Can you work these out from the model? Positions are in its coordinate system, mm. A direction names the side the tool comes from. Give positions to 0.01 mm unless a question says otherwise; leave off trailing zeros. Order: outer loops, then holes, each group sorted by start corner. A loop starts at its lowest first (then second) coordinate and runs counter-clockwise, first axis right, second up. Notation, with made-up numbers: M 43.5,-24 L 69.5,-24 A29 ccw 69.5,1 Z; hole C -25.75,64 d1. An arc over 180 degrees is marked long. Use one line per item in the form item = value. Start each with the question number.
1. I want a section at A-A, the plane z = -35. List the corners of the cut face in (x, y) for me (3 decimals), and give its area (3 significant figures).
2. I want a section at B-B, the plane y = 0.75. List the corners of the cut face in (x, z) for me.
3. For faces 4 (the face through (-9, 1, 3.5)), 5 (the face through (-15, 1, -43)), 6 (the face through (-40, 1, -34)), 7 (the face through (-22, 1, -6)), 8 (the face through (-6, 1, -24)), which set-ups out of +Z, -Z, +X, -X, +Y, -Y let a thin tool reach every point of the face, with its end or its side?
4. I need wall thicknesses on L1, parallel to Z at x = 0, y = 0.9; L2, parallel to Z at x = -3, y = 0.1; L3, parallel to Z at x = -17, y = 1.15. Which ranges of each line are inside material? Lowest first, please.
5. Will these pins go through, and if not, where does the flat tip stop? P1, Ø1.5, axis at x = -24.5, z = -45.5, coming from the -Y side; P2, Ø0.5, axis at y = 1, z = -41, coming from the +X side; P3, Ø0.5, axis at y = 1, z = -8, coming from the -X side.
6. I want a section at C-C, the plane z = -24. List the corners of the cut face in (x, y) for me (3 decimals).
7. We'd pull the mould along X, two halves only. Please class faces 1 (the face through (-39.14, 0.8, -51.6)), 2 (the face through (-18, 0, -24)), 3 (the face through (-11.73, 0.8, -22.78)): +X half, -X half, draft (parallel to the pull), parting line (faces both ways), or undercut.
8. I want a section at D-D, the plane x = -4. List the corners of the cut face in (y, z) for me (3 decimals).
Autodesk Inventor part; units mm, degrees
ref_plane "YZ Plane" through (0, 0, 0) normal (1, 0, 0) x (0, 1, 0)
ref_plane "XZ Plane" through (0, 0, 0) normal (0, 1, 0) x (-1, 0, 0)
ref_plane "XY Plane" through (0, 0, 0) normal (0, 0, 1) x (1, 0, 0)
sketch "Sketch1" plane through (0, 0, 0) normal (0, 1, 0) x (-1, 0, 0)
  circle A0 centre (0, 0) radius 1.3
  circle A1 centre (0, -49) radius 1.3
  arc A2 (0, 3.5) -> (0, -3.5) centre (0, 0) ccw
  arc A3 (0, -45.5) -> (0, -52.5) centre (0, -49) ccw
  line L0 (0, 3.5) -> (19, 3.5)
  line L1 (22, 0.5) -> (22, -13.5)
  line L2 (25, -16.5) -> (37, -16.5)
  line L3 (40, -19.5) -> (40, -49.5)
  line L4 (37, -52.5) -> (0, -52.5)
  line L5 (0, -3.5) -> (3, -3.5)
  line L6 (6, -6.5) -> (6, -42.5)
  line L7 (3, -45.5) -> (0, -45.5)
  arc A4 (6, -6.5) -> (3, -3.5) centre (3, -6.5) ccw
  arc A5 (22, 0.5) -> (19, 3.5) centre (19, 0.5) ccw
  arc A6 (22, -13.5) -> (25, -16.5) centre (25, -13.5) ccw
  arc A7 (40, -19.5) -> (37, -16.5) centre (37, -19.5) ccw
  arc A8 (37, -52.5) -> (40, -49.5) centre (37, -49.5) ccw
  arc A9 (3, -45.5) -> (6, -42.5) centre (3, -42.5) ccw
  circle A10 centre (12, -24) radius 1.25
  circle A11 centre (12, -45.5) radius 1.25
  circle A12 centre (24.5, -45.5) radius 1.25
  circle A13 centre (24.5, -24) radius 1.25
  line L8 (28.5, -30) -> (12, -30)
  line L9 (12, -30) -> (12, -43)
  line L10 (12, -43) -> (19, -43)
  line L11 (19, -43) -> (19, -39.5)
  line L12 (19, -39.5) -> (28.5, -39.5)
  line L13 (28.5, -39.5) -> (28.5, -30)
  line L14 (28.5, -34.75) -> (12, -34.75) construction
  point P0 (22, 3.5)
  point P1 (22, -16.5)
  point P2 (40, -52.5)
  dimension "d0" = 49
  dimension "d1" = 2.6
  dimension "d2" = 7
  dimension "d3" = 22
  dimension "d4" = 20
  dimension "d5" = 40
  dimension "d6" = 6
  dimension "d7" = 3
  dimension "d14" = 2.5
  dimension "d15" = 12.5
  dimension "d16" = 12
  dimension "d17" = 9.5
  dimension "d18" = 3.5
  dimension "d19" = 7
  dimension "d20" = 21.5
  dimension "d21" = 7
extrude "Extrusion1" add sketch "Sketch1" along normal blind 1.615
properties part number "freestanding_cam_mount"
Check result:
q1.outline = M -40,0 L -28.5,0 L -28.5,1.615 L -40,1.615 Z; M -12,0 L -6,0 L -6,1.615 L -12,1.615 Z
q1.area = 28.3 mm2
q2.outline = M -40,-49.5 A3 ccw -37,-52.5 L 0,-52.5 A3.5 ccw 0,-45.5 L -3,-45.5 A3 cw -6,-42.5 L -6,-6.5 A3 cw -3,-3.5 L 0,-3.5 A3.5 ccw 0,3.5 L -19,3.5 A3 ccw -22,0.5 L -22,-13.5 A3 cw -25,-16.5 L -37,-16.5 A3 ccw -40,-19.5 Z; hole M -28.5,-39.5 L -19,-39.5 L -19,-43 L -12,-43 L -12,-30 L -28.5,-30 Z; hole C -24.5,-45.5 d2.5; hole C -24.5,-24 d2.5; hole C -12,-45.5 d2.5; hole C -12,-24 d2.5; hole C 0,-49 d2.6; hole C 0,0 d2.6
q3.face_4 = +Z, +X, -X, +Y, -Y
q3.face_5 = +Y, -Y
q3.face_6 = +Z, -Z, -X, +Y, -Y
q3.face_7 = +Z, -X, +Y, -Y
q3.face_8 = +X, +Y, -Y
q4.L1 = -52.5 to -50.3, -47.7 to -45.5, -3.5 to -1.3, 1.3 to 3.5
q4.L2 = -52.5 to -45.5, -3.5 to 3.5
q4.L3 = -52.5 to -43, -30 to 3.5
q5.P1 = through
q5.P2 = -6
q5.P3 = -22
q6.outline = M -40,0 L -25.75,0 L -25.75,1.615 L -40,1.615 Z; M -23.25,0 L -13.25,0 L -13.25,1.615 L -23.25,1.615 Z; M -10.75,0 L -6,0 L -6,1.615 L -10.75,1.615 Z
q7.face_1 = -X half
q7.face_2 = draft
q7.face_3 = undercut
q8.outline = M 0,-52.5 L 1.615,-52.5 L 1.615,-45.328 L 0,-45.328 Z; M 0,-3.672 L 1.615,-3.672 L 1.615,3.5 L 0,3.5 Z
